Geometry: final body of the model. Coordinates: model frame, mm. A direction names the side the tool comes from. Coordinates: 2 decimals unless noted, no trailing zeros. Order: outer loops, then holes, each group sorted by start corner. A loop starts at its lowest first (then second) coordinate and runs counter-clockwise, first axis right, second up. Notation, with made-up numbers: (81, -40) -> (129, -40) arc R24 cw to (129, -3) -> close; hole circle Ø1 at (-27, 11). An arc over 180 degrees is marked (long way). Answer in a Markdown table with one row per item. Add a question column.
1) Section query A-A on z = 6.5. Return the cut outline in (x, y), then the cut area to 3 significant figures.
2) Pull-direction query (Z, two-part tool) for faces 1 (the face through (28, 4, 7)), 2 (the face through (40, 4, 6)), 3 (the face through (20, 4, 12)); classes: +Z half, -Z half, draft (parallel to the pull), parting line (faces both ways), or undercut.
3) Set-up query: faces 4 (the face through (9.1, 4, 3.9)), 5 (the face through (0, 4, 6)). Return all of +Z, -Z, +X, -X, +Y, -Y with unobstructed straight access to the full face (end or side cutting, diameter ignored); none if empty.
4) Ray query, line 1 (Z direction, x = 31, y = 2.85); line 2 (Z direction, x = 31, y = 7.25); line 3 (X direction, y = 7.25, z = 8.25). Return the intervals inside material, ascending. Write a range as from..to.
5) Section query D-D on x = 10.5. Return the cut outline in (y, z), then the cut area to 3 significant figures.
6) Contact query for flat-ended pins moving along their axis: P1, Ø4, axis at x = 9.5, z = 7.5, coming from the +Y side; P2, Ø4, axis at x = 31, z = 6.5, coming from the -Y side. Output: stop coordinate, or through.
7) Section query B-B on x = 31. Return the cut outline in (y, z), then the cut area to 3 significant figures.
8) Section query C-C on y = 5.25. Return the cut outline in (x, z), then the cut area to 3 significant figures.
```python
from build123d import *

# Parameters (mm, degrees)
SKETCH_1_W                   = 40
SKETCH_1_H                   = 8
EXTRUDE_1_DEPTH              = 12
HOLE_WIZARD_M4_3_D           = 4.8
HOLE_WIZARD_M4_3_CBORE_D     = 8
HOLE_WIZARD_M4_3_CBORE_DEPTH = 4


with BuildPart() as part:
    # 草图1 → 凸台-拉伸1 (new body)
    with BuildSketch(Plane.XY):
        with Locations((20, 4)):
            Rectangle(SKETCH_1_W, SKETCH_1_H)
    extrude(amount=EXTRUDE_1_DEPTH)

    # M4 六角凹头螺钉的柱形沉头孔3 (through all)
    with Locations(Plane(origin=(0, 8, 0), x_dir=(-1, 0, 0), z_dir=(0, 1, 0))):
        with Locations((-9, 6.5), (-31, 6.5)):
            CounterBoreHole(HOLE_WIZARD_M4_3_D / 2, HOLE_WIZARD_M4_3_CBORE_D / 2, HOLE_WIZARD_M4_3_CBORE_DEPTH)


solid = part.part
```
Result:
| question | item | result |
|---|---|---|
| 1 | outline | (0, 0) -> (6.6, 0) -> (6.6, 4) -> (5, 4) -> (5, 8) -> (0, 8) -> close; (11.4, 0) -> (28.6, 0) -> (28.6, 4) -> (27, 4) -> (27, 8) -> (13, 8) -> (13, 4) -> (11.4, 4) -> close; (33.4, 0) -> (40, 0) -> (40, 8) -> (35, 8) -> (35, 4) -> (33.4, 4) -> close |
| 1 | area | 218 mm2 |
| 2 | face 1 | undercut |
| 2 | face 2 | draft |
| 2 | face 3 | +Z half |
| 3 | face 4 | +Y |
| 3 | face 5 | +Z, -Z, -X, +Y, -Y |
| 4 | line 1 | 0..4.1, 8.9..12 |
| 4 | line 2 | 0..2.5, 10.5..12 |
| 4 | line 3 | 0..5.4, 12.6..27.4, 34.6..40 |
| 5 | outline | (0, 0) -> (8, 0) -> (8, 2.79) -> (4, 2.79) -> (4, 4.63) -> (0, 4.63) -> close; (0, 8.37) -> (4, 8.37) -> (4, 10.21) -> (8, 10.21) -> (8, 12) -> (0, 12) -> close |
| 5 | area | 51.3 mm2 |
| 6 | P1 | y = 4 |
| 6 | P2 | through |
| 7 | outline | (0, 0) -> (8, 0) -> (8, 2.5) -> (4, 2.5) -> (4, 4.1) -> (0, 4.1) -> close; (0, 8.9) -> (4, 8.9) -> (4, 10.5) -> (8, 10.5) -> (8, 12) -> (0, 12) -> close |
| 7 | area | 44.8 mm2 |
| 8 | outline | (0, 0) -> (40, 0) -> (40, 12) -> (0, 12) -> close; hole circle Ø8 at (9, 6.5); hole circle Ø8 at (31, 6.5) |
| 8 | area | 379 mm2 |
